```python
from build123d import *

# Parameters (mm, degrees)
F0_W     = 63.5
F0_H     = 50.8
F1_DEPTH = 38.1
F2_R     = 19.05
F3_DEPTH = 25.4
F4_R     = 2.54
F5_T     = -1.27


with BuildPart() as f1:
    # F0 (on Top) → F1 (new body)
    with BuildSketch(Plane.XY):
        with Locations((-3.1476, -8.151593)):
            Rectangle(F0_W, F0_H)
    extrude(amount=F1_DEPTH)

    # F2 (on face) → F3 (cut)
    with BuildSketch(Plane.XY.offset(38.1)):
        with Locations((-3.1476, -8.151593)):
            Circle(F2_R)
    extrude(amount=-F3_DEPTH, mode=Mode.SUBTRACT)

    # F4
    f4_edges = [f1.edges().sort_by_distance(p)[0] for p in [
        (-22.1976, -8.151593, 12.7),
    ]]
    fillet(f4_edges, radius=F4_R)

    # F5
    f5_openings = [f1.faces().sort_by_distance(p)[0] for p in [
        (-3.1476, -8.151593, 0),
    ]]
    offset(amount=F5_T, openings=f5_openings)


solid = f1.part
```
The listing builds one solid part. Answer for the finished solid, in the listing's coordinates (mm). A direction names the side the tool comes from. Coordinates: 2 decimals unless noted, no trailing zeros. Loops run counter-clockwise (first coordinate to the right, second up) from the corner with the lowest first, then second, coordinate; pieces in that order, holes last. Notation, with made-up numbers: (37.5, 51) -> (56.5, 51) arc R23 ccw to (56.5, 65) -> close; hole circle Ø10 at (-10.5, -15). An arc over 180 degrees is marked (long way). Use one line per item in the form item = value. Start each with the question number.
Item 1: The mould has two halves that part along X. Classify faces 1 (the face through (-34, -8, 0)), 2 (the face through (-18.3, -19.7, 26.8)), 3 (the face through (-34.898, -9, 19)), 4 (the face through (28.602, -9, 19)): released by +X, released by -X, zero draft, split by the parting line, or undercut.
Item 2: The part is cut by section A-A on z = 2. Determine the outline of the cut face in (x, y).
Item 3: Consider L1, parallel to X at y = -12, z = 11; L2, parallel to Y at x = -13.5, z = 15.5; L3, parallel to Y at x = -29, z = 20.5. Determine where each line is inside the solid, lowest interval first. Write a range as [from, to].
Item 4: A tool of negligible diameter and unlimited length cuts with its end or side. For faces 5 (the face through (-3, -8, 12.7)), 6 (the face through (27.332, -8, 18)), 7 (the face through (-4, -33.552, 19)), from which of +Z, -Z, +X, -X, +Y, -Y can it reach the whole face along a straight path? Write none if from no direction.
Item 5: Flat-ended cylindrical pins translate along their axes: pin 1 Ø6 at (x, y) = (7, -5) entering from +Z; pin 2 Ø1.5 at (x, y) = (0, -21.5) entering from -Z. Find the tip coordinate at first contact, or state that the pin passes through.
Item 6: The part is cut by section B-B on z = 22. Determine the outline of the cut face in (x, y), then the cut area to 3 significant figures.
Item 7: The part is cut by section C-C on x = 24. Determine the outline of the cut face in (y, z), then the cut area to 3 significant figures.
Answer key:
q1.face_1 = zero draft
q1.face_2 = undercut
q1.face_3 = released by -X
q1.face_4 = released by +X
q2.outline = (-34.9, -33.55) -> (28.6, -33.55) -> (28.6, 17.25) -> (-34.9, 17.25) -> close; hole (-33.63, -32.28) -> (27.33, -32.28) -> (27.33, 15.98) -> (-33.63, 15.98) -> close
q3.L1 = [-34.9, -33.63], [27.33, 28.6]
q3.L2 = [-33.55, -32.28], [-25.64, -24.14], [7.84, 9.33], [15.98, 17.25]
q3.L3 = [-33.55, -32.28], [15.98, 17.25]
q4.face_5 = +Z
q4.face_6 = -Z
q4.face_7 = +Z, -Z, +X, -X, -Y
q5.pin_1 = 12.7
q5.pin_2 = 11.43
q6.outline = (-34.9, -33.55) -> (28.6, -33.55) -> (28.6, 17.25) -> (-34.9, 17.25) -> close; circle Ø40.64 at (-3.15, -8.15); hole (-33.63, -32.28) -> (27.33, -32.28) -> (27.33, 15.98) -> (-33.63, 15.98) -> close; hole circle Ø38.1 at (-3.15, -8.15)
q6.area = 441 mm2
q7.outline = (-33.55, 0) -> (-32.28, 0) -> (-32.28, 36.83) -> (15.98, 36.83) -> (15.98, 0) -> (17.25, 0) -> (17.25, 38.1) -> (-33.55, 38.1) -> close
q7.area = 158 mm2
